Design review of the part built by this model. Coordinates are the model's own, in mm. A direction names the side the tool comes from. Give positions to 0.01 mm unless a question says otherwise; leave off trailing zeros. Order: outer loops, then holes, each group sorted by start corner. A loop starts at its lowest first (then second) coordinate and runs counter-clockwise, first axis right, second up. Notation, with made-up numbers: (81, 72) -> (91, 72) arc R21 cw to (91, 77) -> close; hole circle Ø8 at (-15.5, -13). An arc over 180 degrees is marked (long way). Use a Markdown table: item, result. Add a question column.
```python
from build123d import *

# Parameters (mm, degrees)
EXTRUDE_2_DEPTH     = 50
SKETCH_2_W          = 3
SKETCH_2_H          = 11.5
CUT_EXTRUDE_1_DEPTH = 1.5
FILLET_1_R          = 1.5


with BuildPart() as part:
    # 草图1 → 凸台-拉伸2 (new body)
    with BuildSketch(Plane.XY):
        with BuildLine():
            Line((44.354602366, 43.972629848), (15.854602366, 43.972629848))
            Line((15.854602366, 43.972629848), (-4.145397634, 43.972629848))
            Line((-4.145397634, 43.972629848), (-4.145397634, 45.472629848))
            Line((-4.145397634, 45.472629848), (45.854602366, 45.472629848))
            ThreePointArc((45.854602366, 45.472629848), (46.915262538, 45.03329002), (47.354602366, 43.972629848))
            Line((47.354602366, 43.972629848), (47.354602366, -222.027370152))
            ThreePointArc((47.354602366, -222.027370152), (46.915262538, -223.088030324), (45.854602366, -223.527370152))
            Line((45.854602366, -223.527370152), (14.354602366, -223.527370152))
            Line((14.354602366, -223.527370152), (14.354602366, -212.027370152))
            Line((14.354602366, -212.027370152), (15.854602366, -212.027370152))
            Line((15.854602366, -212.027370152), (15.854602366, -222.027370152))
            Line((15.854602366, -222.027370152), (44.354602366, -222.027370152))
            ThreePointArc((44.354602366, -222.027370152), (45.415262538, -221.588030324), (45.854602366, -220.527370152))
            Line((45.854602366, -220.527370152), (45.854602366, -212.027370152))
            Line((45.854602366, -212.027370152), (45.854602366, -36.027370152))
            Line((45.854602366, -36.027370152), (45.854602366, 42.472629848))
            ThreePointArc((45.854602366, 42.472629848), (45.415262538, 43.53329002), (44.354602366, 43.972629848))
        make_face()
    extrude(amount=EXTRUDE_2_DEPTH)

    # 草图2 → 切除-拉伸1 (cut)
    with BuildSketch(Plane.ZY.offset(-14.354602366)):
        with Locations((48.5, -217.777370152)):
            Rectangle(SKETCH_2_W, SKETCH_2_H)
        with Locations((1.5, -217.777370152)):
            Rectangle(SKETCH_2_W, SKETCH_2_H)
    extrude(amount=-CUT_EXTRUDE_1_DEPTH, mode=Mode.SUBTRACT)

    # 圆角1
    fillet_1_edges = [part.edges().sort_by_distance(p)[0] for p in [
        (14.354602366, -223.527370152, 25),
    ]]
    fillet(fillet_1_edges, radius=FILLET_1_R)


solid = part.part
```
1) For L1, parallel to Y at x = 43, z = 9; L2, parallel to X at y = -26, z = 34.5; L3, parallel to Y at x = 7, z = 21, list the stretches that pass through material, from the lowest coordinate up. Write a range as [from, to].
2) Add section D-D (y = -195). Give the boundary of the cut face in (x, z).
3) The part is to be moulded in two halves that separate along Y. For faces 5 (the flat face through (47, -88, 50)), 6 (the flat face through (31, -223.527, 25)), 7 (the flat face through (30, -222.027, 25)), say which applies: +Y half, -Y half, draft (parallel to the pull), parting line (faces both ways), or undercut.
4) Add section B-B (z = 36.5). Give the boundary of the cut face in (x, y), then the cut area to 3 significant figures.
5) Machinability: for faces 1 (the flat face through (20, 43.973, 25)), 2 (the flat face through (15.855, -217, 25)), 3 (the flat face through (47.355, -87, 25)), 4 (the flat face through (14.355, -217, 25)), which of the approach directions +Z, -Z, +X, -X, +Y, -Y give a long, thin tool a straight path to every point of the face, cutting with its end or side? Answer none if there is none.
6) Add section A-A (x = 25). Give the boundary of the cut face in (y, z), then the cut area to 3 significant figures.
7) Insertion check: pin 1 (1.7 mm diameter, centred on x = 15, y = -216, fed in from +Z); pin 2 (1.6 mm diameter, centred on y = -223, z = 1, fed in from -X); pin 3 (3 mm diameter, centred on y = -216.5, z = 31.5, fed in from -X). Each pin has a flat end and moves straight along its axis. Give the tip position at first contact, or say it passes through.
8) Add section C-C (x = 0.5). Give the boundary of the cut face in (y, z).
Worked answers:
| question | item | result |
|---|---|---|
| 1 | L1 | [-223.53, -222.03], [43.97, 45.47] |
| 1 | L2 | [45.85, 47.35] |
| 1 | L3 | [43.97, 45.47] |
| 2 | outline | (45.85, 0) -> (47.35, 0) -> (47.35, 50) -> (45.85, 50) -> close |
| 3 | face 5 | draft |
| 3 | face 6 | -Y half |
| 3 | face 7 | undercut |
| 4 | outline | (-4.15, 43.97) -> (44.35, 43.97) arc R1.5 cw to (45.85, 42.47) -> (45.85, -220.53) arc R1.5 cw to (44.35, -222.03) -> (15.85, -222.03) -> (15.85, -212.03) -> (14.35, -212.03) -> (14.35, -222.03) arc R1.5 ccw to (15.85, -223.53) -> (45.85, -223.53) arc R1.5 ccw to (47.35, -222.03) -> (47.35, 43.97) arc R1.5 ccw to (45.85, 45.47) -> (-4.15, 45.47) -> close |
| 4 | area | 540 mm^2 |
| 5 | face 1 | +Z, -Z, -X |
| 5 | face 2 | +Z, -Z |
| 5 | face 3 | +Z, -Z, +X, +Y, -Y |
| 5 | face 4 | +Z, -Z, -X, -Y |
| 6 | outline | (-223.53, 0) -> (-222.03, 0) -> (-222.03, 50) -> (-223.53, 50) -> close; (43.97, 0) -> (45.47, 0) -> (45.47, 50) -> (43.97, 50) -> close |
| 6 | area | 150 mm^2 |
| 7 | pin 1 | z = 47 |
| 7 | pin 2 | x = 15.85 |
| 7 | pin 3 | x = 14.35 |
| 8 | outline | (43.97, 0) -> (45.47, 0) -> (45.47, 50) -> (43.97, 50) -> close |
